Here's how the part is built. I have some questions about the finished solid (model axes, mm). Face numbers are marked on the shaded views. A direction names the side the tool comes from. Round coordinates to 2 decimals unless told otherwise and drop trailing zeros. Write each loop counter-clockwise with the first axis right and the second up, starting at its lowest first coordinate (ties: lowest second). Pieces come first, ordered by that corner, then holes. Notation, with made-up numbers: (11.5, -10) -> (26.5, -10) arc R18 ccw to (26.5, 22) -> close; hole circle Ø10 at (67.25, 51). An arc over 180 degrees is marked (long way). Answer in a Markdown table with one row per item. Add a question column.
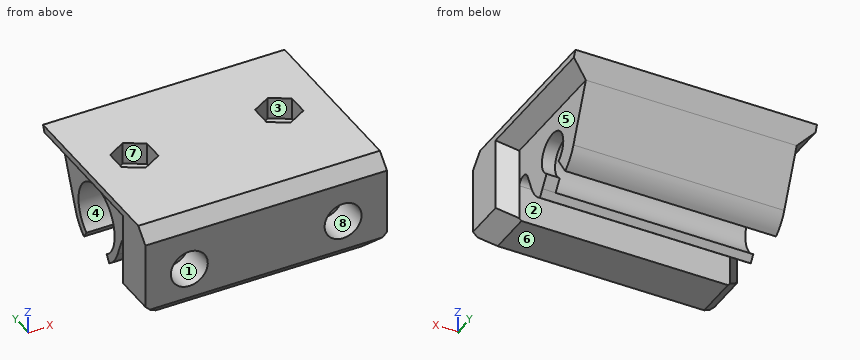
from build123d import *

# Parameters (mm, degrees)
SKETCH1_W           = 55
SKETCH1_H           = 45
BOSS_EXTRUDE1_DEPTH = 5
SKETCH3_W           = 55
SKETCH3_H           = 13
BOSS_EXTRUDE5_DEPTH = 20
CHAMFER1_SIZE       = 3
SKETCH5_R           = 4.2
CUT_EXTRUDE2_DEPTH  = 8
BOSS_EXTRUDE7_DEPTH = 48
CUT_EXTRUDE3_DEPTH  = 71.205777697
CHAMFER2_SIZE       = 3.5
CHAMFER3_SIZE       = 3.5
CHAMFER4_SIZE       = 7
BOSS_EXTRUDE8_START = -3
BOSS_EXTRUDE8_DEPTH = 3
CHAMFER5_SIZE       = 6
CUT_EXTRUDE4_DEPTH  = 5
SKETCH11_W          = 55
SKETCH11_H          = 13.699454105
CUT_EXTRUDE5_DEPTH  = 3


with BuildPart() as part:
    # Sketch1 → Boss-Extrude1 (new body)
    with BuildSketch(Plane.XY):
        with Locations((17.145774036, 16.279520652)):
            Rectangle(SKETCH1_W, SKETCH1_H)
    extrude(amount=BOSS_EXTRUDE1_DEPTH)

    # Sketch3 → Boss-Extrude5 (add)
    with BuildSketch(Plane(origin=(0, 0, 0), x_dir=(-1, 0, 0), z_dir=(0, 0, -1))):
        with Locations((-17.145774036, 0.279520652)):
            Rectangle(SKETCH3_W, SKETCH3_H)
    extrude(amount=BOSS_EXTRUDE5_DEPTH)

    # Chamfer1
    chamfer1_edges = [part.edges().sort_by_distance(p)[0] for p in [
        (17.145774036, -6.220479348, 5),
    ]]
    chamfer(chamfer1_edges, length=CHAMFER1_SIZE)

    # Sketch5 → Cut-Extrude2 (cut)
    with BuildSketch(Plane.XZ.offset(6.220479348)):
        with Locations(Location((-0.354225964, -7, 0), (0, 0, 270))):
            Circle(SKETCH5_R)
        with Locations(Location((34.645774036, -7, 0), (0, 0, 270))):
            Circle(SKETCH5_R)
    extrude(amount=-CUT_EXTRUDE2_DEPTH, mode=Mode.SUBTRACT)

    # Sketch7 → Boss-Extrude7 (add)
    with BuildSketch(Plane.ZY.offset(6.854225964)):
        with BuildLine():
            Line((-8.308177677, 10.21387745), (-12.629175087, 12.000050953))
            ThreePointArc((-12.629175087, 12.000050953), (-15.003318067, 13.416764905), (-16.86901604, 15.457060078))
            Line((-16.86901604, 15.457060078), (-15.295212832, 16.521552193))
            ThreePointArc((-15.295212832, 16.521552193), (-1.4, 20.779520652), (-15.295212832, 25.037489111))
            Line((-15.295212832, 25.037489111), (-16.86901604, 26.101981226))
            ThreePointArc((-16.86901604, 26.101981226), (-15.003318067, 28.142276398), (-12.629175087, 29.55899035))
            Line((-12.629175087, 29.55899035), (0, 34.779520652))
            Line((0, 34.779520652), (0, 6.779520652))
            Line((0, 6.779520652), (-8.576470695, 6.779520652))
            ThreePointArc((-8.576470695, 6.779520652), (-7.194534972, 8.39922137), (-8.308177677, 10.21387745))
        make_face()
    extrude(amount=-BOSS_EXTRUDE7_DEPTH)

    # Sketch8 → Cut-Extrude3 (cut, through all)
    with BuildSketch(Plane.ZY.offset(10.354225964)):
        Polygon((0, 34.779520652), (5, 36.846373896), (5, 38.779520652), (0, 38.779520652), align=None)
    extrude(amount=-CUT_EXTRUDE3_DEPTH, mode=Mode.SUBTRACT)

    # Chamfer2
    chamfer2_edges = [part.edges().sort_by_distance(p)[0] for p in [
        (-10.354225964, 6.779520652, -10),
        (-10.354225964, 20.779520652, 0),
    ]]
    chamfer(chamfer2_edges, length=CHAMFER2_SIZE - 0.0001)  # a hair under: the kernel refuses the full size

    # Chamfer3
    chamfer3_edges = [part.edges().sort_by_distance(p)[0] for p in [
        (44.645774036, 20.779520652, 0),
        (44.645774036, 6.779520652, -10),
    ]]
    chamfer(chamfer3_edges, length=CHAMFER3_SIZE - 0.0001)  # a hair under: the kernel refuses the full size

    # Chamfer4
    chamfer4_edges = [part.edges().sort_by_distance(p)[0] for p in [
        (44.645774036, -1.470429348, -20),
        (-10.354225964, -1.470429348, -20),
    ]]
    chamfer(chamfer4_edges, length=CHAMFER4_SIZE)

    # Sketch9 → Boss-Extrude8 (add)
    with BuildSketch(Plane(origin=(41.145774036, 0, 0), x_dir=(0, 0, -1), z_dir=(1, 0, 0)).offset(BOSS_EXTRUDE8_START)):
        with BuildLine():
            Line((15.295212832, 16.521552193), (12.727428651, 18.258355117))
            ThreePointArc((12.727428651, 18.258355117), (4.5, 20.779520652), (12.727428651, 23.300686187))
            Line((12.727428651, 23.300686187), (15.295212832, 25.037489111))
            ThreePointArc((15.295212832, 25.037489111), (1.4, 20.779520652), (15.295212832, 16.521552193))
        make_face()
    extrude(amount=BOSS_EXTRUDE8_DEPTH)

    # Chamfer5
    chamfer5_edges = [part.edges().sort_by_distance(p)[0] for p in [
        (17.145774036, -6.220479348, -20),
    ]]
    chamfer(chamfer5_edges, length=CHAMFER5_SIZE)

    # Sketch10 → Cut-Extrude4 (cut)
    with BuildSketch(Plane.XY.offset(5)):
        Polygon((33.645774036, 13.92977839), (37.845774036, 16.354649521), (37.845774036, 21.204391782), (33.645774036, 23.629262913), (29.445774036, 21.204391782), (29.445774036, 16.354649521), align=None)
        Polygon((0.645774036, 13.92977839), (4.845774036, 16.354649521), (4.845774036, 21.204391782), (0.645774036, 23.629262913), (-3.554225964, 21.204391782), (-3.554225964, 16.354649521), align=None)
    extrude(amount=-CUT_EXTRUDE4_DEPTH, mode=Mode.SUBTRACT)

    # Sketch11 → Cut-Extrude5 (cut)
    with BuildSketch(Plane(origin=(0, 0, -20), x_dir=(-1, 0, 0), z_dir=(0, 0, -1))):
        with Locations((-17.145774036, 0.629247705)):
            Rectangle(SKETCH11_W, SKETCH11_H)
    extrude(amount=-CUT_EXTRUDE5_DEPTH, mode=Mode.SUBTRACT)


solid = part.part
Item 1: I need wall thicknesses on line 1 along X through (y, z) = (-3, -7); line 2 along Y through (x, z) = (34, -8.75); line 3 along X through (y, z) = (-0.5, -6.5). Which ranges of each line are inside material? Lowest first, please. Write a range as from..to.
Item 2: If we mould it in two halves opening along Z, with no side actions, what happens to the marked faces 6, 7 and 8? For each: pulls with the +Z half, pulls with the -Z half, needs draft (parallel to the pull), parting line crosses it, or undercut.
Item 3: On a 3-axis mill with a long thin cutter (end or side, diameter ignored), from which of +Z, -Z, +X, -X, +Y, -Y can I reach the whole of each face in a straight line? I mean the marked faces 1, 2, 3, 4 and 5. Say none if no direction works.
Item 4: If we section it at D-D on x = 36: Please give me the cut outline in (y, z).
Item 5: If we section it at B-B on x = 23: Please give me the cut outline in (y, z).
Item 6: For P1, Ø11, axis at x = -0.35, z = -7, coming from the +Y side; P2, Ø5, axis at y = 22, z = -11, coming from the -X side; P3, Ø8, axis at y = 31.5, z = -4.5, coming from the -X side, each with a flat end and sliding along its axis, tell me the tip position at first contact or that it passes through.
Results list:
| question | item | result |
|---|---|---|
| 1 | line 1 | -10.35..-4.55, 3.85..30.45, 38.85..44.65 |
| 1 | line 2 | 1.78..6.78, 10.4..13.18, 28.38..31.16 |
| 1 | line 3 | -10.35..-4.52, 3.82..30.48, 38.82..44.65 |
| 2 | face 6 | pulls with the -Z half |
| 2 | face 7 | needs draft |
| 2 | face 8 | undercut |
| 3 | face 1 | -Y |
| 3 | face 2 | -Z, +X, -X |
| 3 | face 3 | +Z |
| 3 | face 4 | -X |
| 3 | face 5 | -Z, +X, +Y |
| 4 | outline | (-6.22, -14) -> (-3.22, -17) -> (6.78, -17) -> (6.78, -8.58) arc R1.81 cw to (10.21, -8.31) -> (12, -12.63) arc R9.5 ccw to (15.46, -16.87) -> (16.52, -15.3) arc R7.6 cw (long way) to (25.04, -15.3) -> (26.1, -16.87) arc R9.5 ccw to (29.56, -12.63) -> (36.85, 5) -> (22.27, 5) -> (22.27, 0) -> (15.29, 0) -> (15.29, 5) -> (-3.22, 5) -> (-6.22, 2) -> (-6.22, -3.02) -> (1.78, -3.02) -> (1.78, -10.98) -> (-6.22, -10.98) -> close |
| 5 | outline | (-6.22, -14) -> (-3.22, -17) -> (6.78, -17) -> (6.78, -8.58) arc R1.81 cw to (10.21, -8.31) -> (12, -12.63) arc R9.5 ccw to (15.46, -16.87) -> (16.52, -15.3) arc R7.6 cw (long way) to (25.04, -15.3) -> (26.1, -16.87) arc R9.5 ccw to (29.56, -12.63) -> (36.85, 5) -> (-3.22, 5) -> (-6.22, 2) -> close |
| 6 | P1 | y = 34.16 |
| 6 | P2 | x = 38.15 |
| 6 | P3 | x = -6.85 |
